Verification items for the finished model (mm, model axes). Face numbers are marked on the shaded views. A direction names the side the tool comes from. Round coordinates to 2 decimals unless told otherwise and drop trailing zeros. Order: outer loops, then holes, each group sorted by start corner. A loop starts at its lowest first (then second) coordinate and runs counter-clockwise, first axis right, second up. Notation, with made-up numbers: (79.5, 52.5) -> (124.5, 52.5) arc R32 ccw to (124.5, 86.5) -> close; hole circle Ø5 at (63, 49.5). An arc over 180 degrees is marked (long way). Return JSON: item names as keys, results as strings. Group by question number.
Item 1: Access from +Z, -Z, +X, -X, +Y, -Y to the whole of each face (thin tool, end or side, straight path). Record for the marked faces 1 and 2.
Item 2: Sectioned sample at B-B on z = 9. Record the cut outline in (x, y), plus the area to 3 significant figures.
Item 3: Depth check by flat-ended pin: pin 1 Ø4.5 at (y, z) = (3.5, 3) entering from +X; pin 2 Ø1.5 at (x, y) = (85.5, 22.5) entering from +Z; pin 3 Ø6 at (x, y) = (96, -6) entering from -Z; pin 4 Ø4.5 at (x, z) = (34.5, 2) entering from +Y. Enter the tip coordinate at first touch or a pass-through.
Item 4: Scan lines: probe 1 along Z at (x, y) = (34.5, 2); probe 2 along Y at (x, z) = (96, 3.05); probe 3 along Y at (x, z) = (19, 3). Record each from-to range of solid material in increasing order. Write a range as from..to.
Item 5: Sectioned sample at A-A on x = 39.5. Record the cut outline in (y, z), plus the area to 3 significant figures.
```python
from build123d import *

# Parameters (mm, degrees)
SKETCH1_R           = 5
BOSS_EXTRUDE1_DEPTH = 4
BOSS_EXTRUDE2_START = -65.921828
BOSS_EXTRUDE2_DEPTH = 65.921828
FILLET1_R           = 12


with BuildPart() as part:
    # Sketch1 → Boss-Extrude1 (new body)
    with BuildSketch(Plane.XY):
        with BuildLine():
            Line((0, 0), (0, 34))
            ThreePointArc((0, 34), (3.514718626, 42.485281374), (12, 46))
            Line((12, 46), (54, 46))
            Line((54, 46), (108, 8.188792937))
            Line((108, 8.188792937), (108, -6))
            ThreePointArc((108, -6), (104.485281374, -14.485281374), (96, -18))
            Line((96, -18), (18, -18))
            Line((18, -18), (0, 0))
        make_face()
        with Locations((12, 34)):
            Circle(SKETCH1_R, mode=Mode.SUBTRACT)
        with Locations((96, -6)):
            Circle(SKETCH1_R, mode=Mode.SUBTRACT)
    extrude(amount=BOSS_EXTRUDE1_DEPTH)

    # Sketch5 → Boss-Extrude2 (add)
    with BuildSketch(Plane(origin=(68.621613592, -48.049371121, 0), x_dir=(0, 0, -1), z_dir=(0.819152044288997, -0.5735764363510386, 0)).offset(BOSS_EXTRUDE2_START)):
        with BuildLine():
            Line((-4, 68.6541216), (0, 68.6541216))
            Line((0, 68.6541216), (0, 79.44625787))
            Line((0, 79.44625787), (-16.501573626, 86.113326382))
            Line((-16.501573626, 86.113326382), (-18, 82.404590964))
            Line((-18, 82.404590964), (-11.504720879, 79.780327855))
            ThreePointArc((-11.504720879, 79.780327855), (-6.051549129, 75.364436442), (-4, 68.6541216))
        make_face()
    extrude(amount=BOSS_EXTRUDE2_DEPTH)

    # Fillet1
    fillet1_edges = [part.edges().sort_by_distance(p)[0] for p in [
        (87.190114977, 35.934797015, 0),
    ]]
    fillet(fillet1_edges, radius=FILLET1_R)


solid = part.part
```
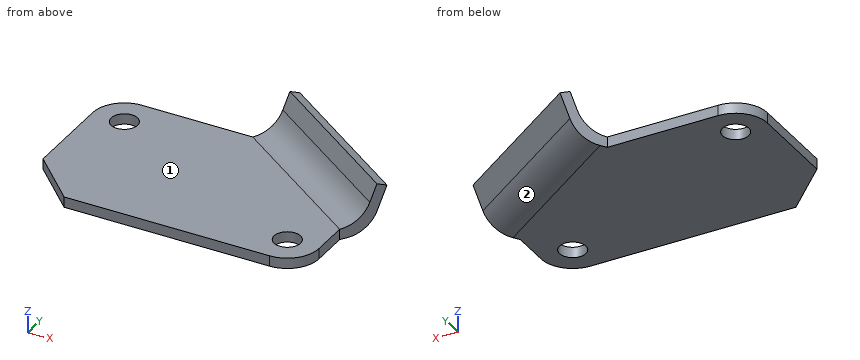
Recorded:
{
 "1": {"face 1": "+Z, -X, -Y", "face 2": "-Z, +X, +Y"},
 "2": {"outline": "(59.59, 53.98) -> (113.59, 16.17) -> (116.28, 20.01) -> (62.28, 57.82) -> close", "area": "309 mm²"},
 "3": {"pin 1": "x = 108", "pin 2": "z = 4", "pin 3": "through", "pin 4": "y = 46"},
 "4": {"probe 1": "0..4", "probe 2": "-18..-11, -1..29.64", "probe 3": "-18..46"},
 "5": {"outline": "(-18, 0) -> (46, 0) -> (46, 4) -> (-18, 4) -> close", "area": "256 mm²"}
}
